Autodesk Inventor part; units mm, degrees
ref_plane "YZ Plane" through (0, 0, 0) normal (1, 0, 0) x (0, 1, 0)
ref_plane "XZ Plane" through (0, 0, 0) normal (0, 1, 0) x (-1, 0, 0)
ref_plane "XY Plane" through (0, 0, 0) normal (0, 0, 1) x (1, 0, 0)
sketch "Sketch1" plane through (0, 0, 0) normal (0, 0, 1) x (1, 0, 0)
  line L0 (0, 0) -> (6.45, 0)
  line L1 (6.45, 0) -> (6.45, 5)
  line L2 (6.45, 5) -> (6.9597, 5)
  line L3 (7.3939, 4.7479) -> (8.2527, 3.2437)
  line L4 (8.2527, 1.7563) -> (7.3939, 0.2521)
  line L5 (6.9597, 0) -> (6.45, 0)
  arc A0 (8.2527, 1.7563) -> (8.2527, 3.2437) centre (6.95, 2.5) ccw
  arc A1 (7.3939, 4.7479) -> (6.9597, 5) centre (6.9597, 4.5) ccw
  arc A2 (6.9597, 0) -> (7.3939, 0.2521) centre (6.9597, 0.5) ccw
  line L6 (0, 0) -> (0, 12.2617)
  point P0 (7.25, 5)
  point P1 (7.25, 0)
  dimension "d0" = 5
  dimension "d1" = 6.45
  dimension "d2" = 0.8
  dimension "d3" = 1.5
  dimension "d4" = 0.5
  dimension "d5" = 2
revolve "Revolution1" add sketch "Sketch1" angle 360 about axis through (0, 0, 0) along (0, 1, 0)
chamfer "Chamfer1" distance 0.1 angle 45 2 edges at (-6.45, 0, 0) (-6.45, 5, 0)
properties part number "idl-tire"
Geometry: final body of the model. Coordinates: model frame, mm. Coordinates: 2 decimals unless noted, no trailing zeros. Order: outer loops, then holes, each group sorted by start corner. A loop starts at its lowest first (then second) coordinate and runs counter-clockwise, first axis right, second up.
1) Ray query, probe 1 along Z at (x, y) = (0.75, 0.65); probe 2 along Z at (x, y) = (0, 1.8); probe 3 along X at (y, z) = (1.95, -1.25). Return the intervals inside material, ascending.
Result sheet:
probe 1: z = -7.58 to -6.41, 6.41 to 7.58
probe 2: z = -8.28 to -6.45, 6.45 to 8.28
probe 3: x = -8.25 to -6.33, 6.33 to 8.25
2) Section A-A (z = 0). Return loops of the section in (x, y).
Result sheet:
outline: (-8.25, 1.76) - (-7.39, 0.25) arc R0.5 ccw to (-6.96, 0) - (-6.55, 0) - (-6.45, 0.1) - (-6.45, 4.9) - (-6.55, 5) - (-6.96, 5) arc R0.5 ccw to (-7.39, 4.75) - (-8.25, 3.24) arc R1.5 ccw to start; (6.45, 0.1) - (6.55, 0) - (6.96, 0) arc R0.5 ccw to (7.39, 0.25) - (8.25, 1.76) arc R1.5 ccw to (8.25, 3.24) - (7.39, 4.75) arc R0.5 ccw to (6.96, 5) - (6.55, 5) - (6.45, 4.9) - close
3) Section C-C (y = 2). Return loops of the section in (x, z), then the cut area to 3 significant figures.
Result sheet:
outline: circle Ø16.73 at (0, 0); hole circle Ø12.9 at (0, 0)
area: 89.1 mm2
4) Section B-B (x = 0). Return loops of the section in (y, z), then the cut area to 3 significant figures.
Result sheet:
outline: (0, -6.96) arc R0.5 ccw to (0.25, -7.39) - (1.76, -8.25) arc R1.5 ccw to (3.24, -8.25) - (4.75, -7.39) arc R0.5 ccw to (5, -6.96) - (5, -6.55) - (4.9, -6.45) - (0.1, -6.45) - (0, -6.55) - close; (0, 6.55) - (0.1, 6.45) - (4.9, 6.45) - (5, 6.55) - (5, 6.96) arc R0.5 ccw to (4.75, 7.39) - (3.24, 8.25) arc R1.5 ccw to (1.76, 8.25) - (0.25, 7.39) arc R0.5 ccw to (0, 6.96) - close
area: 14.8 mm2
5) Draft query along Z for faces 1 (the flat face through (3, 5, 6)), 2 (the cylindrical face through (-1.398, 2.534, 6.297)). Return one class per face: released by +Z, released by -Z, zero draft, split by the parting line, or undercut.
Result sheet:
face 1: zero draft
face 2: undercut
6) First-contact query: P1, Ø2, axis at x = 4, y = 1.5, coming from the +Z side; P2, Ø2, axis at y = 2, z = -2.5, coming from the +X side; P3, Ø8, axis at x = 2.5, z = -6, coming from the +Y side; P4, Ø6, axis at x = -3, z = -1.5, coming from the +Y side. Flat tips, straight axial feed; report the tip coordinate or a pass-through.
Result sheet:
P1: stops at z = 7.76
P2: stops at x = 8.3
P3: stops at y = 5
P4: passes through
7) Section D-D (y = 0.6). Return loops of the section in (x, z).
Result sheet:
outline: circle Ø15.19 at (0, 0); hole circle Ø12.9 at (0, 0)
